from build123d import *

# Parameters (mm, degrees)
F0_W     = 12.7
F0_H     = 12.7
F1_DEPTH = 203.2
F3_DEPTH = 25.4
F4_W     = 9.7917
F4_H     = 9.7917
F5_DEPTH = 254
F6_R     = 2.38125
F7_DEPTH = 25.4


with BuildPart() as f1:
    # F0 (on Top) → F1 (new body)
    with BuildSketch(Plane.XY):
        with Locations((6.35, 6.35)):
            Rectangle(F0_W, F0_H)
    extrude(amount=F1_DEPTH)

    # F2 (on face) → F3 (cut)
    with BuildSketch(Plane.XZ):
        with BuildLine():
            ThreePointArc((0, 10.998523), (0, -10.998523), (19.05, 0))
            ThreePointArc((19.05, 0), (17.348523, 6.35), (12.7, 10.998523))
            Line((12.7, 10.998523), (12.7, 0))
            Line((12.7, 0), (0, 0))
            Line((0, 0), (0, 10.998523))
        make_face()
        with BuildLine():
            Line((12.7, 0), (12.7, 10.998523))
            ThreePointArc((12.7, 10.998523), (6.35, 12.7), (0, 10.998523))
            Line((0, 10.998523), (0, 0))
            Line((0, 0), (12.7, 0))
        make_face()
    extrude(amount=-F3_DEPTH, mode=Mode.SUBTRACT)

    # F4 (on face) → F5 (cut)
    with BuildSketch(Plane.XY.offset(203.2)):
        with Locations((6.35, 6.35)):
            Rectangle(F4_W, F4_H)
    extrude(amount=-F5_DEPTH, mode=Mode.SUBTRACT)

    # F6 (on face) → F7 (cut)
    with BuildSketch(Plane.XZ):
        with Locations((6.35, 50.8)):
            Circle(F6_R)
    extrude(amount=-F7_DEPTH, mode=Mode.SUBTRACT)


solid = f1.part
The model under review builds one solid part; all positions refer to its coordinate system, in mm. A direction names the side the tool comes from. Round coordinates to 2 decimals unless told otherwise and drop trailing zeros. Write each loop counter-clockwise with the first axis right and the second up, starting at its lowest first coordinate (ties: lowest second). Pieces come first, ordered by that corner, then holes. Notation, with made-up numbers: M 27.5,5.25 L 68.5,5.25 A22 ccw 68.5,43.25 Z; hole C 50.25,47.5 d8. An arc over 180 degrees is marked long. Use a Markdown table: item, result. Add a question column.
Q1. Machinability: for faces 5 (the face through (6.04, 11.96, 53.16)), 6 (the face through (11.246, 6, 109)), which of the approach directions +Z, -Z, +X, -X, +Y, -Y give a long, thin tool a straight path to every point of the face, cutting with its end or side? Answer none if there is none.
Q2. We need section C-C, the plane x = 6.35. State the section outline as (y, z) points.
Q3. The part is to be moulded in two halves that separate along X. For faces 1 (the face through (12.7, 6, 106)), 2 (the face through (0, 6, 106)), 3 (the face through (6, 1.454, 109)), 4 (the face through (1.454, 6, 109)), say which applies: pulls with the +X half, pulls with the -X half, needs draft (parallel to the pull), parting line crosses it, or undercut.
Q4. To check wall thickness, follow line 1 (Y direction, x = 8, z = 125); line 2 (Z direction, x = 6.35, y = 11.85). State the ranges of each line that lie inside material, in increasing order.
Q5. We need section B-B, the plane y = 4.75. State the section outline as (x, z) points.
Q6. We need section A-A, the plane z = 63. State the section outline as (x, y) points, plus the area to 3 significant figures.
Findings below:
| question | item | result |
|---|---|---|
| 1 | face 5 | +Y, -Y |
| 1 | face 6 | +Z, -Z |
| 2 | outline | M 0,12.7 L 1.45,12.7 L 1.45,48.42 L 0,48.42 Z; M 0,53.18 L 1.45,53.18 L 1.45,203.2 L 0,203.2 Z; M 11.25,12.7 L 12.7,12.7 L 12.7,48.42 L 11.25,48.42 Z; M 11.25,53.18 L 12.7,53.18 L 12.7,203.2 L 11.25,203.2 Z |
| 3 | face 1 | pulls with the +X half |
| 3 | face 2 | pulls with the -X half |
| 3 | face 3 | undercut |
| 3 | face 4 | undercut |
| 4 | line 1 | y = 0 to 1.45, 11.25 to 12.7 |
| 4 | line 2 | z = 12.7 to 48.42, 53.18 to 203.2 |
| 5 | outline | M 0,11 A12.7 cw 1.45,11.72 L 1.45,203.2 L 0,203.2 Z; M 11.25,11.72 A12.7 cw 12.7,11 L 12.7,203.2 L 11.25,203.2 Z |
| 6 | outline | M 0,0 L 12.7,0 L 12.7,12.7 L 0,12.7 Z; hole M 1.45,1.45 L 11.25,1.45 L 11.25,11.25 L 1.45,11.25 Z |
| 6 | area | 65.4 mm² |
